Autodesk Fusion 360 part; units mm, degrees
sketch "Sketch1" plane through (0, 0, 0) normal (0, 0, 1) x (1, 0, 0) in component "Halterung"
  line L0 (0, 0) -> (29, 0)
  line L1 (29, 0) -> (29, 29)
  line L2 (29, 29) -> (0, 29)
  line L3 (0, 29) -> (0, 0)
  circle A0 centre (7.5, 7.5) radius 3.5
  circle A1 centre (21.5, 7.5) radius 3.5
  circle A2 centre (7.5, 21.5) radius 3.5
  circle A3 centre (21.5, 21.5) radius 3.5
  dimension "d1" = 7
  dimension "d3" = 4
  dimension "d6" = 7
  dimension "d7" = 4
  dimension "d8" = 7
  dimension "d9" = 4
  dimension "d10" = 4
  dimension "d15" = 35
extrude "Extrude1" add sketch "Sketch1" along normal blind 60 in component "Halterung"
sketch "Sketch2" plane through (0, 29, 0) normal (0, 1, 0) x (-1, 0, 0) in component "Halterung"
  line L0 (-29, 0) -> (0, 0)
  line L1 (0, 0) -> (0, 60)
  line L2 (0, 60) -> (-29, 60)
  line L3 (-29, 60) -> (-29, 0)
  line L4 (-29, 60) -> (-26, 60)
  line L5 (-26, 60) -> (-26, 40)
  line L6 (-26, 40) -> (-29, 40)
  line L7 (-29, 40) -> (-29, 60)
  line L8 (-14.5, 60) -> (-14.5, 0) construction
  line L9 (-3, 60) -> (-3, 40)
  line L10 (0, 60) -> (-3, 60)
  line L11 (0, 40) -> (0, 60)
  line L12 (-3, 40) -> (0, 40)
  dimension "d13" = 3
  dimension "d14" = 20
extrude "Extrude2" add sketch "Sketch2" along normal blind 56.5 contours L2 L3 L4 L5 L6 L7 | L1 L2 L9 L10 L11 L12 in component "Halterung"
sketch "Sketch3" plane through (29, 0, 0) normal (1, 0, 0) x (0, 1, 0) in component "Halterung"
  line L0 (0, 0) -> (29, 0)
  line L1 (29, 0) -> (29, 40)
  line L2 (29, 40) -> (85.5, 40)
  line L3 (85.5, 40) -> (85.5, 60)
  line L4 (85.5, 60) -> (0, 60)
  line L5 (0, 60) -> (0, 0)
  line L6 (85.5, 60) -> (81.5, 60)
  line L7 (81.5, 60) -> (81.5, 40)
  line L8 (81.5, 40) -> (85.5, 40)
  line L9 (85.5, 40) -> (85.5, 60)
  dimension "d18" = 4
extrude "Extrude3" add sketch "Sketch3" along normal blind 16 contours L2 L3 L4 L6 L7 L8 L9 in component "Halterung"
extrude "Extrude4" add sketch "Sketch3" against normal blind 16 from surface at -29 contours L2 L3 L4 L6 L7 L8 L9 in component "Halterung"
sketch "Sketch4" plane through (0, 81.5, 0) normal (0, -1, 0) x (1, 0, 0) in component "Halterung"
  line L0 (29, 60) -> (29, 40)
  line L1 (29, 40) -> (45, 40)
  line L2 (45, 40) -> (45, 60)
  line L3 (45, 60) -> (29, 60)
  circle A0 centre (37, 50) radius 5.5
  line L4 (45, 50) -> (29, 50) construction
  line L5 (37, 60) -> (37, 40) construction
  line L6 (14.5, 0) -> (14.5, 60) construction
  line L7 (0, 60) -> (29, 60)
  line L8 (0, 0) -> (29, 0)
  circle A1 centre (37, 50) radius 2.75
  circle A2 centre (-8, 50) radius 5.5
  circle A3 centre (-8, 50) radius 2.75
  point P0 (37, 50)
  dimension "d24" = 11
  dimension "d25" = 5.5
extrude "Extrude5" cut sketch "Sketch4" against normal up to surface (4 mm away) contours A1 | A3 in component "Halterung"
extrude "Extrude6" cut sketch "Sketch4" against normal blind 2 contours A0 | A2 in component "Halterung"
sketch "Sketch1 (2)" plane through (0, 0, 0) normal (0, 0, -1) x (1, 0, 0)
  line L0 (0, 0) -> (0, -29)
  line L1 (0, -29) -> (29, -29)
  line L2 (29, -29) -> (29, 0)
  line L3 (29, 0) -> (0, 0)
  circle A0 centre (7.5, -7.5) radius 2.9
  circle A1 centre (21.5, -7.5) radius 2.9
  circle A2 centre (7.5, -21.5) radius 2.9
  circle A3 centre (21.5, -21.5) radius 2.9
  circle A4 centre (21.5, -21.5) radius 3.5
  circle A5 centre (7.5, -21.5) radius 3.5
  circle A6 centre (21.5, -7.5) radius 3.5
  circle A7 centre (7.5, -7.5) radius 3.5
  dimension "d52" = 5.8
extrude "Extrude9" add sketch "Sketch1 (2)" against normal blind 5 contours A4 | A5 | A6 | A7 in component "Halterung"
chamfer "Chamfer2" distance 3 angle 45 4 edges at (4.7963, 20.4513, 0) (18.7963, 20.4513, 0) (18.7963, 6.4513, 0) (4.7963, 6.4513, 0) in component "Halterung"
component "Halterung" placed x (1, 0, 0) y (0, 1, 0) z (0, 0, 1) at (0, 0, 0)
Geometry: final body of the model. Coordinates: model frame, mm. A direction names the side the tool comes from. Coordinates: 2 decimals unless noted, no trailing zeros. Order: outer loops, then holes, each group sorted by start corner. A loop starts at its lowest first (then second) coordinate and runs counter-clockwise, first axis right, second up. Notation, with made-up numbers: (63, 71) - (81, 71) arc R16 cw to (81, 86) - close; hole circle Ø5 at (71, -30). An arc over 180 degrees is marked (long way). Return JSON: item names as keys, results as strings. Group by question number.
1. Set-up query: faces 5 (the face through (33, 81.5, 55)), 6 (the face through (36.284, 82.486, 55.453)), 7 (the face through (1, 65, 40)). Return all of +Z, -Z, +X, -X, +Y, -Y with unobstructed straight access to the full face (end or side cutting, diameter ignored); none if empty.
2. Cut plane C-C (y = 80). Output: boundary loops of the cut face in (x, z).
3. Cut plane B-B (z = 50). Count the separate pieces of the cut face and the enclosed holes in it, plus the area to 3 significant figures.
4. Cut plane A-A (x = 7.5). Output: boundary loops of the cut face in (y, z), plus the area to 3 significant figures.
5. Material intervals for line 1 along Y through (x, z) = (21.5, 27.5); line 2 along Y through (x, z) = (21.5, 4.3), sorted ascending. Write a range as [from, to].
6. Pull-direction query (X, two-part tool) for faces 1 (the face through (28, 65, 40)), 2 (the face through (4.003, 7.346, 32.115)), 3 (the face through (20.831, 24.514, 2.812)), 4 (the face through (0, 32, 43)); classes: pulls with the +X half, pulls with the -X half, needs draft (parallel to the pull), parting line crosses it, or undercut.
7. Pin query (flat end, axial travel): pin 1 (8.5 mm diameter, centred on x = 13.5, z = 28, fed in from +Y); pin 2 (8 mm diameter, centred on y = 28, z = 39.5, fed in from +X); pin 3 (3.5 mm diameter, centred on x = 7, y = 8, fed in from +Z); pin 4 (11 mm diameter, centred on x = 7.5, y = 21.5, fed in from -Z). Return the tip coordinate at first contact, or that it passes through.
Resolved:
{
 "1": {"face 5": "+Z, -Z, +X, -Y", "face 6": "-Y", "face 7": "-Z, +X, -X, +Y"},
 "2": {"outline": "(0, 40) - (3, 40) - (3, 60) - (0, 60) - close; (26, 40) - (29, 40) - (29, 60) - (26, 60) - close"},
 "3": {"separate pieces": "3", "enclosed holes": "4", "area": "1,090 mm²"},
 "4": {"outline": "(0, 0) - (1.6, 0) - (4.6, 3) - (4.6, 5) - (4, 5) - (4, 60) - (0, 60) - close; (10.4, 3) - (13.4, 0) - (15.6, 0) - (18.6, 3) - (18.6, 5) - (18, 5) - (18, 60) - (11, 60) - (11, 5) - (10.4, 5) - close; (24.4, 3) - (27.4, 0) - (29, 0) - (29, 60) - (25, 60) - (25, 5) - (24.4, 5) - close", "area": "894 mm²"},
 "5": {"line 1": "y = [0, 4], [11, 18], [25, 29]", "line 2": "y = [0, 4.6], [10.4, 18.6], [24.4, 29]"},
 "6": {"face 1": "needs draft", "face 2": "undercut", "face 3": "undercut", "face 4": "pulls with the -X half"},
 "7": {"pin 1": "stops at y = 29", "pin 2": "stops at x = 29", "pin 3": "passes through", "pin 4": "stops at z = 0.4"}
}
